Build history of the part. All positions in model axes, mm. Round coordinates to 2 decimals unless told otherwise and drop trailing zeros. Write each loop counter-clockwise with the first axis right and the second up, starting at its lowest first coordinate (ties: lowest second). Pieces come first, ordered by that corner, then holes. Notation, with made-up numbers: (33, 40) - (78, 40) arc R17 cw to (78, 63) - close; hole circle Ø8 at (20.5, 36.5). An arc over 180 degrees is marked (long way). Answer as a JSON object with one key per item and string values. Group by question number.
Item 1: Slice it at B-B, the plane y = -35. List the corners of the cut face in (x, z).
Item 2: Probe line 1 (Y direction, x = 65, z = -3.4); line 2 (Y direction, x = 80, z = -2.15); line 3 (X direction, y = 12.5, z = -5.7). List the from-to ranges inside material, lowest first. Write a range as from..to.
Item 3: Slice it at A-A, the plane x = 80. List the corners of the cut face in (y, z).
Item 4: Slice it at D-D, the plane x = -65. List the corners of the cut face in (y, z), then the cut area to 3 significant figures.
Item 5: Slice it at C-C, the plane z = -5. List the corners of the cut face in (x, y).
Item 6: Flat gauge pin, fed straight in: pin 1 (3.5 mm diameter, centred on x = -80, y = -55, fed in from +Z). Where does the tip first touch, or does it go through?
from build123d import *

# Parameters (mm, degrees)
SKETCH_W     = 200
SKETCH_H     = 150
PAD_DEPTH    = 6
FILLET_R     = 3
SKETCH001_R  = 2.75
SKETCH001_W  = 90
SKETCH001_H  = 42
POCKET_DEPTH = 6.001


with BuildPart() as part:
    # Sketch → Pad (new body)
    with BuildSketch(Plane.XY):
        Rectangle(SKETCH_W, SKETCH_H)
    extrude(amount=-PAD_DEPTH)

    # Fillet
    fillet_edges = [part.edges().sort_by_distance(p)[0] for p in [
        (-100, -75, -3),
        (100, -75, -3),
        (100, 75, -3),
        (-100, 75, -3),
    ]]
    fillet(fillet_edges, radius=FILLET_R)

    # Sketch001 (on Face2 of Fillet) → Pocket (cut, through all)
    with BuildSketch(Plane.XY):
        with Locations((-80, -55)):
            Circle(SKETCH001_R)
        with Locations((80, -55)):
            Circle(SKETCH001_R)
        with Locations((-65, 47)):
            Circle(SKETCH001_R)
        with Locations((65, 47)):
            Circle(SKETCH001_R)
        with Locations((65, -35)):
            Circle(SKETCH001_R)
        with Locations((-65, -35)):
            Circle(SKETCH001_R)
        with Locations((0, 6)):
            Rectangle(SKETCH001_W, SKETCH001_H)
    extrude(amount=-POCKET_DEPTH, mode=Mode.SUBTRACT)


solid = part.part
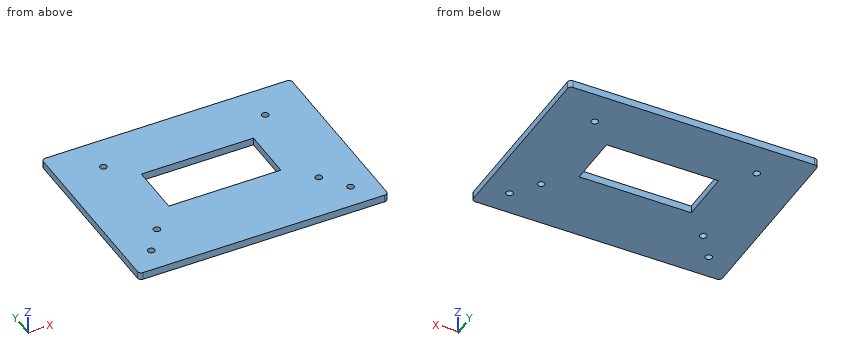
Geometry says:
{
 "1": {"outline": "(-100, -6) - (-67.75, -6) - (-67.75, 0) - (-100, 0) - close; (-62.25, -6) - (62.25, -6) - (62.25, 0) - (-62.25, 0) - close; (67.75, -6) - (100, -6) - (100, 0) - (67.75, 0) - close"},
 "2": {"line 1": "y = -75..-37.75, -32.25..44.25, 49.75..75", "line 2": "y = -75..-57.75, -52.25..75", "line 3": "x = -100..-45, 45..100"},
 "3": {"outline": "(-75, -6) - (-57.75, -6) - (-57.75, 0) - (-75, 0) - close; (-52.25, -6) - (75, -6) - (75, 0) - (-52.25, 0) - close"},
 "4": {"outline": "(-75, -6) - (-37.75, -6) - (-37.75, 0) - (-75, 0) - close; (-32.25, -6) - (44.25, -6) - (44.25, 0) - (-32.25, 0) - close; (49.75, -6) - (75, -6) - (75, 0) - (49.75, 0) - close", "area": "834 mm^2"},
 "5": {"outline": "(-100, -72) arc R3 ccw to (-97, -75) - (97, -75) arc R3 ccw to (100, -72) - (100, 72) arc R3 ccw to (97, 75) - (-97, 75) arc R3 ccw to (-100, 72) - close; hole circle Ø5.5 at (-80, -55); hole circle Ø5.5 at (-65, -35); hole circle Ø5.5 at (-65, 47); hole (-45, -15) - (45, -15) - (45, 27) - (-45, 27) - close; hole circle Ø5.5 at (65, -35); hole circle Ø5.5 at (65, 47); hole circle Ø5.5 at (80, -55)"},
 "6": {"pin 1": "passes through"}
}
